```python
from build123d import *

# Parameters (mm, degrees)
ESQUISSE1_W                = 200
ESQUISSE1_H                = 40
BOSS_EXTRU_1_DEPTH         = 6
ENL_V_MAT_EXTRU_1_DEPTH    = 103.156742313
ESQUISSE3_R                = 2.5
ENL_V_MAT_EXTRU_2_DEPTH    = 103.156742313
R_P_TITION_LIN_AIRE1_COUNT = 12
R_P_TITION_LIN_AIRE1_PITCH = 16


with BuildPart() as part:
    # Esquisse1 → Boss.-Extru.1 (new body)
    with BuildSketch(Plane.XY):
        Rectangle(ESQUISSE1_W, ESQUISSE1_H)
    extrude(amount=BOSS_EXTRU_1_DEPTH)

    # Esquisse2 → Enlèv. mat.-Extru.1 (cut, through all)
    with BuildSketch(Plane.XY.offset(6)):
        with BuildLine():
            Line((-92.8, 14.4), (-92.8, 20))
            Line((-92.8, 20), (-83.2, 20))
            Line((-83.2, 20), (-83.2, 14.4))
            ThreePointArc((-83.2, 14.4), (-88, 8), (-92.8, 14.4))
        make_face()
    enl_v_mat_extru_1 = extrude(amount=-ENL_V_MAT_EXTRU_1_DEPTH, mode=Mode.SUBTRACT)

    # Esquisse3 → Enlèv. mat.-Extru.2 (cut, through all)
    with BuildSketch(Plane.XY.offset(6)):
        with Locations((-85, -5)):
            Circle(ESQUISSE3_R)
        with Locations((85, -5)):
            Circle(ESQUISSE3_R)
        with Locations((0, -5)):
            Circle(ESQUISSE3_R)
    extrude(amount=-ENL_V_MAT_EXTRU_2_DEPTH, mode=Mode.SUBTRACT)

    # Répétition linéaire1: Enlèv. mat.-Extru.1 ×12
    with Locations(*[(i * R_P_TITION_LIN_AIRE1_PITCH, 0, 0) for i in range(1, R_P_TITION_LIN_AIRE1_COUNT)]):
        add(enl_v_mat_extru_1, mode=Mode.SUBTRACT)


solid = part.part
```
The listing builds one solid part. Answer for the finished solid, in the listing's coordinates (mm). A direction names the side the tool comes from. Round coordinates to 2 decimals unless told otherwise and drop trailing zeros. Write each loop counter-clockwise with the first axis right and the second up, starting at its lowest first coordinate (ties: lowest second). Pieces come first, ordered by that corner, then holes. Notation, with made-up numbers: (37.25, -20.75) -> (74.25, -20.75) arc R9 cw to (74.25, -5.75) -> close; hole circle Ø3 at (22.25, 19.25). An arc over 180 degrees is marked (long way). Write item = value, one per line.
1) Section D-D on x = 85 is taken. Write down the section's boundary in (y, z).
Check values:
outline = (-20, 0) -> (-7.5, 0) -> (-7.5, 6) -> (-20, 6) -> close; (-2.5, 0) -> (9, 0) -> (9, 6) -> (-2.5, 6) -> close
2) Section A-A on x = 0 is taken. Write down the section's boundary in (y, z), plus the area to 3 significant figures.
Check values:
outline = (-20, 0) -> (-7.5, 0) -> (-7.5, 6) -> (-20, 6) -> close; (-2.5, 0) -> (20, 0) -> (20, 6) -> (-2.5, 6) -> close
area = 210 mm²
3) For a pull along X with two mould halves and no side action, classify faces 1 (the flat face through (-80, 20, 3)), 2 (the flat face through (100, 0, 3)), 3 (the cylindrical face through (-8, 8, 3)) as released by +X, released by -X, zero draft, split by the parting line, or undercut.
Check values:
face_1 = zero draft
face_2 = released by +X
face_3 = undercut
4) Given pin 1 (5 mm diameter, centred on x = -6.5, y = 2, fed in from -Z), flat-ended and moving along its own axis, determine where the tip first touches the part or whether it passes through.
Check values:
pin_1 = 0
5) Which of the six approach directions +Z, -Z, +X, -X, +Y, -Y give full straight-line access (tool end or side, diameter ignored) to faces 4 (the flat face through (67.2, 17, 3)), 5 (the flat face through (32, 20, 3))?
Check values:
face_4 = +Z, -Z, +Y
face_5 = +Z, -Z, +X, -X, +Y
6) Section B-B on z = 2.2 is taken. Give the number of separate pieces and of enclosed holes in the cut face, plus the area to 3 significant figures.
Check values:
separate_pieces = 1
enclosed_holes = 3
area = 6,660 mm²
7) Straight lines are drawn through the part: line 1 along Y through (x, z) = (0, 3.75); line 2 along Y through (x, z) = (88, 3.6); line 3 along Y through (x, z) = (-1.5, 5.6). For each, find the intervals that lie inside material, in ascending order. Write a range as [from, to].
Check values:
line_1 = [-20, -7.5], [-2.5, 20]
line_2 = [-20, 8]
line_3 = [-20, -7], [-3, 20]
